Read the model definition and answer for the solid it produces. Units are mm, in the model's axes. Face numbers are marked on the shaded views. A direction names the side the tool comes from. Give positions to 0.01 mm unless a question says otherwise; leave off trailing zeros. Order: outer loops, then holes, each group sorted by start corner. A loop starts at its lowest first (then second) coordinate and runs counter-clockwise, first axis right, second up. Notation, with made-up numbers: M 4.25,55 L 61.25,55 A30 ccw 61.25,92 Z; hole C 71,30 d2. An arc over 180 degrees is marked long. One line per item, written item: value.
from build123d import *

# Parameters (mm, degrees)
SKETCH_1_R                   = 20
EXTRUDE_1_DEPTH              = 17.5
HOLE_WIZARD_M6_1_D           = 8
HOLE_WIZARD_M6_1_CBORE_D     = 14
HOLE_WIZARD_M6_1_CBORE_DEPTH = 6
HOLE_WIZARD_M5_1_D           = 4.2
HOLE_WIZARD_M5_1_DEPTH       = 12.4
HOLE_WIZARD_M5_1_TIP         = 1.2618073
CUT_EXTRUDE_2_REACH          = 85.08
CUT_EXTRUDE_2_END_RADIUS     = 20
SKETCH_5_R                   = 5


with BuildPart() as part:
    # 草图1 → 拉伸1 (new, symmetric)
    with BuildSketch(Plane.XY):
        Polygon((30, 14), (50, 14), (50, 0), (-50, 0), (-50, 14), (-30, 14), (-30, 59), (-25, 64), (25, 64), (30, 59), align=None)
        with Locations((0, 33)):
            Circle(SKETCH_1_R, mode=Mode.SUBTRACT)
    extrude(amount=EXTRUDE_1_DEPTH, both=True)

    # M6 六角凹头螺钉的柱形沉头孔1 (through all)
    with Locations(Plane(origin=(-40, 14, 10), x_dir=(0, 0, 1), z_dir=(0, 1, 0))):
        with Locations((0, 0), (-20, 0), (-20, 80), (0, 80)):
            CounterBoreHole(HOLE_WIZARD_M6_1_D / 2, HOLE_WIZARD_M6_1_CBORE_D / 2, HOLE_WIZARD_M6_1_CBORE_DEPTH)

    # M5 螺纹孔1
    with Locations(Plane(origin=(-17.67766953, 15.32233047, 17.5), x_dir=(1, 0, 0), z_dir=(0, 0, 1))):
        with Locations((0, 0), (35.35533906, 0), (35.35533906, 35.35533906), (0, 35.35533906)):
            Hole(HOLE_WIZARD_M5_1_D / 2, depth=HOLE_WIZARD_M5_1_DEPTH)
            with Locations((0, 0, -(HOLE_WIZARD_M5_1_DEPTH + HOLE_WIZARD_M5_1_TIP / 2))):  # 118° drill point
                Cone(0, HOLE_WIZARD_M5_1_D / 2, HOLE_WIZARD_M5_1_TIP, mode=Mode.SUBTRACT)

    # 拉伸2: up to this cylinder (the profile starts outside it)
    cut_extrude_2_end = Plane(origin=(0, 33, -5), z_dir=(0, 0, -1)) * Cylinder(CUT_EXTRUDE_2_END_RADIUS, 211.16, mode=Mode.PRIVATE)
    # 草图5 → 拉伸2 (cut, up to the surface)
    with BuildSketch(Plane(origin=(0, 64, 0), x_dir=(1, 0, 0), z_dir=(0, 1, 0)), mode=Mode.PRIVATE) as cut_extrude_2_sk1:
        with Locations(Location((0, 5, 0), (0, 0, 270))):
            Circle(SKETCH_5_R)
    cut_extrude_2_tool1 = extrude(cut_extrude_2_sk1.sketch, amount=-CUT_EXTRUDE_2_REACH, mode=Mode.PRIVATE) - cut_extrude_2_end
    add(cut_extrude_2_tool1.solids().sort_by_distance((0, 64, -5))[0], mode=Mode.SUBTRACT)


solid = part.part
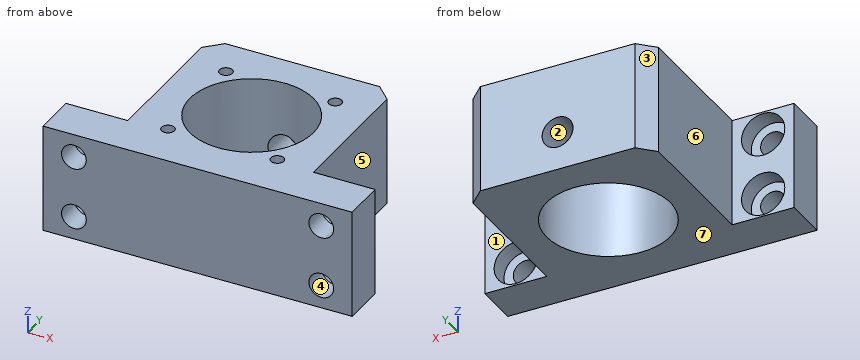
1) Find section D-D, the plane x = 0. Write down the section's boundary in (y, z).
Reported:
outline: M 0,-17.5 L 13,-17.5 L 13,17.5 L 0,17.5 Z; M 53,-17.5 L 64,-17.5 L 64,-10 L 53,-10 Z; M 53,0 L 64,0 L 64,17.5 L 53,17.5 Z
2) Each of these flat-tipped pins is pushed along its axis until it touches: pin 1 Ø3 at (y, z) = (22, -12) entering from +X; pin 2 Ø2 at (y, z) = (21, 13.5) entering from -X; pin 3 Ø11 at (x, z) = (38, -13) entering from +Y. Where does it stop, or does it pass through?
Reported:
pin 1: stops at x = 30
pin 2: stops at x = -30
pin 3: stops at y = 14
3) Find section C-C, the plane z = 10. Count the separate pieces of the cut face and the enclosed holes in it, plus the area to 3 significant figures.
Reported:
separate pieces: 3
enclosed holes: 5
area: 2,770 mm^2
4) Which of the six approach directions +Z, -Z, +X, -X, +Y, -Y give full straight-line access (tool end or side, diameter ignored) to the marked faces 5, 6 and 7?
Reported:
face 5: +Z, -Z, +X, +Y
face 6: +Z, -Z, -X, +Y
face 7: -Z, +X, -X, +Y, -Y
5) Determine the mould class of the marked faces 1, 2, 3 and 4 for opening direction X: +X half, -X half, draft (parallel to the pull), parting line (faces both ways), or undercut.
Reported:
face 1: draft
face 2: undercut
face 3: -X half
face 4: undercut
6) Find section A-A, the plane x = -40. Write down the section's boundary in (y, z).
Reported:
outline: M 0,-17.5 L 14,-17.5 L 14,-17 L 8,-17 L 8,-14 L 0,-14 Z; M 0,-6 L 8,-6 L 8,-3 L 14,-3 L 14,3 L 8,3 L 8,6 L 0,6 Z; M 0,14 L 8,14 L 8,17 L 14,17 L 14,17.5 L 0,17.5 Z
7) Consider probe 1 along X at (y, z) = (12.45, -10); probe 2 along Z at (x, y) = (0, 57.75); probe 3 along Z at (x, y) = (41.5, 10). Determine where each line is inside the solid, lowest interval first.
Reported:
probe 1: x = -50 to -47, -33 to 33, 47 to 50
probe 2: z = -17.5 to -10, 0 to 17.5
probe 3: z = -17.5 to -16.84, -3.16 to 3.16, 16.84 to 17.5
8) Find section B-B, the plane y = 21. Write down the section's boundary in (x, z).
Reported:
outline: M -30,-17.5 L -16,-17.5 L -16,17.5 L -30,17.5 Z; M 16,-17.5 L 30,-17.5 L 30,17.5 L 16,17.5 Z
